Autodesk Inventor part; units mm, degrees
ref_plane "YZ Plane" through (0, 0, 0) normal (1, 0, 0) x (0, 1, 0)
ref_plane "XZ Plane" through (0, 0, 0) normal (0, 1, 0) x (-1, 0, 0)
ref_plane "XY Plane" through (0, 0, 0) normal (0, 0, 1) x (1, 0, 0)
sketch "Sketch1" plane through (0, 0, 0) normal (0, 0, 1) x (1, 0, 0)
  circle A0 centre (0, 0) radius 4
  circle A1 centre (0, 0) radius 14.5
  line L0 (-27.5, -14.5) -> (27.5, -14.5)
  line L1 (27.5, -14.5) -> (27.5, -9.31)
  line L2 (27.5, -9.31) -> (-27.5, -9.31)
  line L3 (-27.5, -9.31) -> (-27.5, -14.5)
  dimension "d0" = 8
  dimension "d1" = 29
  dimension "d2" = 27.5
  dimension "d3" = 27.5
  dimension "d4" = 5.19
extrude "Extrusion1" add sketch "Sketch1" along normal blind 13
sketch "Sketch2" plane through (11.1164, -9.31, 0) normal (0, 1, 0) x (1, 0, 0)
  line L0 (-22.2328, -13) -> (-22.2328, 0)
  line L1 (-22.2328, 0) -> (-38.6164, 0)
  line L2 (-38.6164, 0) -> (-38.6164, -13)
  line L3 (-22.2328, -13) -> (-38.6164, -13)
  line L4 (0, 0) -> (0, -13)
  line L5 (16.3836, -13) -> (0, -13)
  line L6 (16.3836, 0) -> (16.3836, -13)
  line L7 (16.3836, 0) -> (0, 0)
  circle A0 centre (-32.1164, -6.5) radius 2.5
  circle A1 centre (9.8836, -6.5) radius 2.5
  line L8 (0, 0) -> (0, -13)
  line L9 (-22.2328, 0) -> (0, 0)
  line L10 (-22.2328, -13) -> (-22.2328, 0)
  line L11 (0, -13) -> (-22.2328, -13)
  point P0 (-11.1164, 0)
  dimension "d7" = 5
  dimension "d8" = 5
  dimension "d9" = 21
  dimension "d10" = 21
extrude "Extrusion2" cut sketch "Sketch2" against normal through all contours A0 | A1
chamfer "Chamfer1" distance 2 angle 45 4 edges at (-27.5, -11.905, 0) (27.5, -11.905, 0) (27.5, -11.905, 13) (-27.5, -11.905, 13)
properties part number "00_spindel_bearings"
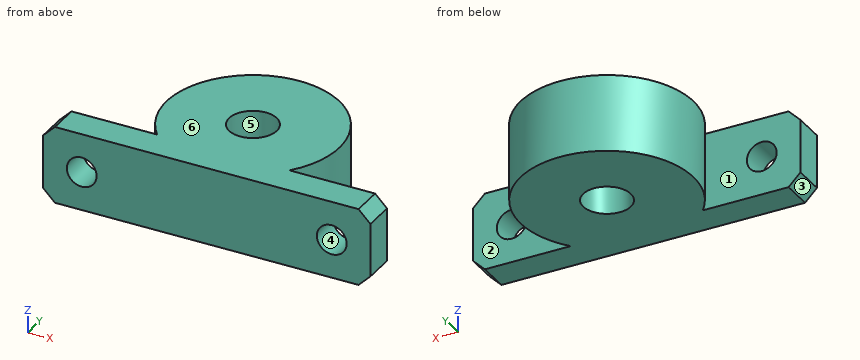
Read the model definition and answer for the solid it produces. Units are mm, in the model's axes. Face numbers are marked on the shaded views. A direction names the side the tool comes from. Coordinates: 2 decimals unless noted, no trailing zeros. Order: outer loops, then holes, each group sorted by start corner. A loop starts at its lowest first (then second) coordinate and runs counter-clockwise, first axis right, second up. Notation, with made-up numbers: (-4, 22.25) - (25, 22.25) arc R21 cw to (25, 28.25) - close; hole circle Ø5 at (21, 9). An arc over 180 degrees is marked (long way). Answer as a JSON object with one key per item and string values. Group by question number.
Item 1: Flat-ended cylindrical pins translate along their axes: P1, Ø4, axis at x = 22.5, z = 6.5, coming from the +Y side; P2, Ø10, axis at x = 6.5, y = 1, coming from the -Z side; P3, Ø3, axis at x = -21, z = 6.5, coming from the -Y side; P4, Ø1.5, axis at y = -5.5, z = 10.5, coming from the +X side. Find the tip coordinate at first contact, or state that the pin passes through.
Item 2: Section B-B (y = -12.5) is taken. Give the vertices of the cut face in (x, z).
Item 3: A tool of negligible diameter and unlimited length cuts with its end or side. For the marked faces 1, 2 and 3, from which of +Z, -Z, +X, -X, +Y, -Y can it reach the whole face along a straight path? Write none if from no direction.
Item 4: Consider probe 1 along X at (y, z) = (-11.95, 6.5); probe 2 along Z at (x, y) = (21, -13.25); probe 3 along X at (y, z) = (1.25, 6.5). Determine where each line is inside the solid, lowest interval first. Write a range as from..to.
Item 5: Section A-A (z = 6.5) is taken. Give the vertices of the cut face in (x, y), plus the area to 3 significant figures.
Item 6: Section C-C (x = 0) is taken. Give the vertices of the cut face in (y, z).
Item 7: The mould has two halves that part along Z. Classify the marked faces 4, 5 and 6: +Z half, -Z half, draft (parallel to the pull), parting line (faces both ways), or undercut.
Results are:
{
 "1": {"P1": "stops at y = -9.31", "P2": "stops at z = 0", "P3": "passes through", "P4": "stops at x = 13.7"},
 "2": {"outline": "(-27.5, 2) - (-25.5, 0) - (25.5, 0) - (27.5, 2) - (27.5, 11) - (25.5, 13) - (-25.5, 13) - (-27.5, 11) - close; hole circle Ø5 at (-21, 6.5); hole circle Ø5 at (21, 6.5)"},
 "3": {"face 1": "+Z, -Z, -X", "face 2": "+Z, -Z, +X", "face 3": "-Z, -X, +Y, -Y"},
 "4": {"probe 1": "x = -27.5..-23.5, -18.5..18.5, 23.5..27.5", "probe 2": "z = 0..4, 9..13", "probe 3": "x = -14.45..-3.8, 3.8..14.45"},
 "5": {"outline": "(-27.5, -14.5) - (-23.5, -14.5) - (-23.5, -9.31) - (-27.5, -9.31) - close; (-18.5, -14.5) - (18.5, -14.5) - (18.5, -9.31) - (11.12, -9.31) arc R14.5 ccw (long way) to (-11.12, -9.31) - (-18.5, -9.31) - close; (23.5, -14.5) - (27.5, -14.5) - (27.5, -9.31) - (23.5, -9.31) - close; hole circle Ø8 at (0, 0)", "area": "764 mm^2"},
 "6": {"outline": "(-14.5, 0) - (-4, 0) - (-4, 13) - (-14.5, 13) - close; (4, 0) - (14.5, 0) - (14.5, 13) - (4, 13) - close"},
 "7": {"face 4": "undercut", "face 5": "draft", "face 6": "+Z half"}
}
